For this review, take the finished solid that the model builds, in its own axes (mm). Coordinates: 2 decimals unless noted, no trailing zeros. Loops run counter-clockwise (first coordinate to the right, second up) from the corner with the lowest first, then second, coordinate; pieces in that order, holes last. Notation, with made-up numbers: (-16.75, -37.75) - (17.25, -37.75) arc R27 cw to (17.25, -20.75) - close; hole circle Ø5 at (62.5, 67.25). An arc over 180 degrees is marked (long way). Answer as a JSON object with one key per item and string values. Group by question number.
Item 1: We need section A-A (y = 0). Give the boundary of the cut face in (x, z).
Item 2: We need section C-C (z = 2.5). Give the boundary of the cut face in (x, y).
Item 3: To check wall thickness, follow line 1 (Y direction, x = 0, z = 1.3); line 2 (Y direction, x = -14, z = 1); line 3 (X direction, y = 14.5, z = 6). State the ranges of each line that lie inside material, in increasing order.
Item 4: Clearance check with flat-ended pins moving along their axes: pin 1 (3 mm diameter, centred on y = -23.5, z = 1.5, fed in from -X); pin 2 (1.5 mm diameter, centred on y = 88.5, z = 3.5, fed in from +X); pin 3 (3 mm diameter, centred on x = -49.5, z = 4.5, fed in from +Y). State where each tip first meets the part, or that it passes through.
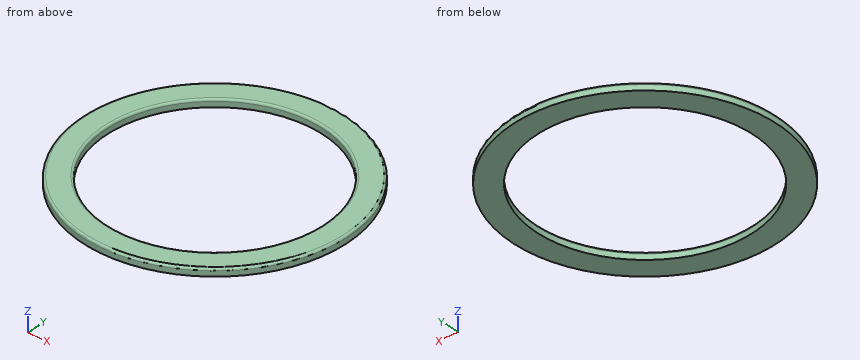
from build123d import *

# Parameters (mm, degrees)
F0_R     = 122.5
F1_DEPTH = 7
F2_R     = 100.5
F3_DEPTH = 25
F4_R     = 2


with BuildPart() as f1:
    # F0 (on Top) → F1 (new body)
    with BuildSketch(Plane.XY):
        Circle(F0_R)
    extrude(amount=F1_DEPTH)

    # F2 (on face) → F3 (cut)
    with BuildSketch(Plane.XY.offset(7)):
        Circle(F2_R)
    extrude(amount=-F3_DEPTH, mode=Mode.SUBTRACT)

    # F4
    f4_edges = [f1.edges().sort_by_distance(p)[0] for p in [
        (-122.5, 0, 7),
        (-100.5, 0, 7),
    ]]
    fillet(f4_edges, radius=F4_R)


solid = f1.part
Check sheet entries:
{
 "1": {"outline": "(-122.5, 0) - (-100.5, 0) - (-100.5, 5) arc R2 ccw to (-102.5, 7) - (-120.5, 7) arc R2 ccw to (-122.5, 5) - close; (100.5, 0) - (122.5, 0) - (122.5, 5) arc R2 ccw to (120.5, 7) - (102.5, 7) arc R2 ccw to (100.5, 5) - close"},
 "2": {"outline": "circle Ø245 at (0, 0); hole circle Ø201 at (0, 0)"},
 "3": {"line 1": "y = -122.5 to -100.5, 100.5 to 122.5", "line 2": "y = -121.7 to -99.52, 99.52 to 121.7", "line 3": "x = -121.37 to -99.72, 99.72 to 121.37"},
 "4": {"pin 1": "stops at x = -120.51", "pin 2": "stops at x = 85.48", "pin 3": "stops at y = 112.7"}
}
